```python
from build123d import *

# Parameters (mm, degrees)
SKETCH2_R               = 18
BOSS_EXTRUDE1_DEPTH     = 60
BOSS_EXTRUDE2_DEPTH     = 53
BOSS_EXTRUDE3_DEPTH     = 2
CUT_EXTRUDE3_DEPTH      = 97.822001632
CUT_EXTRUDE3_DEPTH_BACK = 97.822001632
BOSS_EXTRUDE4_START     = -56
SKETCH6_R               = 18
BOSS_EXTRUDE4_DEPTH     = 56
SKETCH8_R               = 3.017040472
BOSS_EXTRUDE5_DEPTH     = 10
SKETCH9_R               = 40
BOSS_EXTRUDE6_DEPTH     = 4.2
CUT_EXTRUDE4_DEPTH      = 104.317471969
CIRPATTERN1_COUNT       = 3


with BuildPart() as part:
    # Sketch2 → Boss-Extrude1 (new body)
    with BuildSketch(Plane.XY):
        Circle(SKETCH2_R)
    extrude(amount=BOSS_EXTRUDE1_DEPTH)

    # Sketch3 → Boss-Extrude2 (add)
    with BuildSketch(Plane.XY):
        with BuildLine():
            Line((-25.5, 0), (-25.5, 58.5))
            Line((-25.5, 58.5), (25.5, 58.5))
            Line((25.5, 58.5), (25.5, 0))
            ThreePointArc((25.5, 0), (0, -25.5), (-25.5, 0))
        make_face()
    extrude(amount=BOSS_EXTRUDE2_DEPTH)

    # Sketch4 → Boss-Extrude3 (add)
    with BuildSketch(Plane.XY):
        with BuildLine():
            Line((-3.6, 19.027416998), (-19.027416998, 3.6))
            Line((-19.027416998, 3.6), (-44.9, 3.6))
            ThreePointArc((-44.9, 3.6), (-48.5, 0), (-44.9, -3.6))
            Line((-44.9, -3.6), (-19.027416998, -3.6))
            Line((-19.027416998, -3.6), (-3.6, -19.027416998))
            Line((-3.6, -19.027416998), (-3.6, -44.9))
            ThreePointArc((-3.6, -44.9), (0, -48.5), (3.6, -44.9))
            Line((3.6, -44.9), (3.6, -19.027416998))
            Line((3.6, -19.027416998), (19.027416998, -3.6))
            Line((19.027416998, -3.6), (44.9, -3.6))
            ThreePointArc((44.9, -3.6), (48.5, 0), (44.9, 3.6))
            Line((44.9, 3.6), (19.027416998, 3.6))
            Line((19.027416998, 3.6), (3.6, 19.027416998))
            Line((3.6, 19.027416998), (3.6, 44.9))
            ThreePointArc((3.6, 44.9), (0, 48.5), (-3.6, 44.9))
            Line((-3.6, 44.9), (-3.6, 19.027416998))
        make_face()
    extrude(amount=-BOSS_EXTRUDE3_DEPTH)

    # Sketch5 → Cut-Extrude3 (cut, two sides: drawn at the far end of the back side and taken through both)
    with BuildSketch(Plane(origin=(0, 0, 0), x_dir=(0, 0, -1), z_dir=(1, 0, 0)).offset(-CUT_EXTRUDE3_DEPTH_BACK)):
        with BuildLine():
            Line((-53, 14.147312787), (-45.647312787, 14.147312787))
            ThreePointArc((-45.647312787, 14.147312787), (-17.612429059, 2.534883727), (-6, -25.5))
            Line((-6, -25.5), (-53, -25.5))
            Line((-53, -25.5), (-53, 14.147312787))
        make_face()
    extrude(amount=CUT_EXTRUDE3_DEPTH + CUT_EXTRUDE3_DEPTH_BACK, mode=Mode.SUBTRACT)

    # Sketch6 → Boss-Extrude4 (add)
    with BuildSketch(Plane.XY.offset(60).offset(BOSS_EXTRUDE4_START)):
        with Locations(Location((0, 0, 0), (0, 0, 128.190277301))):
            Circle(SKETCH6_R)
    extrude(amount=BOSS_EXTRUDE4_DEPTH)

    # Sketch8 → Boss-Extrude5 (add)
    with BuildSketch(Plane.XY):
        Circle(SKETCH8_R)
    extrude(amount=-BOSS_EXTRUDE5_DEPTH)

    # Sketch9 → Boss-Extrude6 (add)
    with BuildSketch(Plane(origin=(0, 0, -10), x_dir=(-1, 0, 0), z_dir=(0, 0, -1))):
        Circle(SKETCH9_R)
    extrude(amount=BOSS_EXTRUDE6_DEPTH)

    # Sketch11 → Cut-Extrude4 (cut, through all)
    with BuildSketch(Plane.XY.offset(-10)):
        with BuildLine():
            Line((12.5, 0), (30, 0))
            ThreePointArc((30, 0), (19.283628291, 22.981333294), (-5.20944533, 29.54423259))
            Line((-5.20944533, 29.54423259), (-2.170602221, 12.310096913))
            ThreePointArc((-2.170602221, 12.310096913), (8.034845121, 9.575555539), (12.5, 0))
        make_face()
    cut_extrude4 = extrude(amount=-CUT_EXTRUDE4_DEPTH, mode=Mode.SUBTRACT)

    # CirPattern1: Cut-Extrude4 ×3 about axis
    cirpattern1_axis = Axis((0, 0, 0), (0, 0, 1))
    for i in range(1, CIRPATTERN1_COUNT):
        add(cut_extrude4.rotate(cirpattern1_axis, i * 360 / CIRPATTERN1_COUNT), mode=Mode.SUBTRACT)


solid = part.part
```
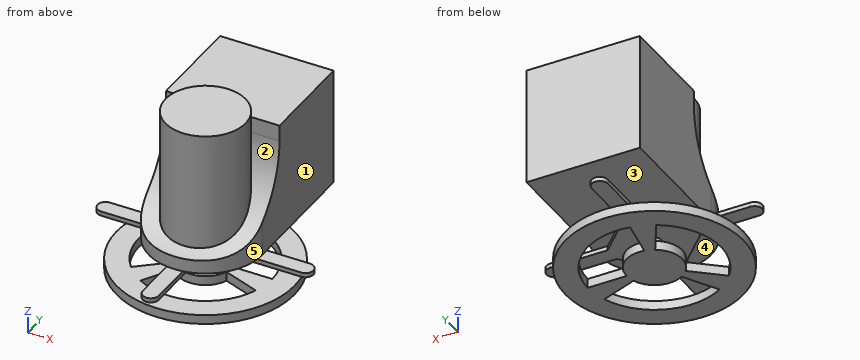
Design review of the part built by this model. Coordinates are the model's own, in mm. Face numbers are marked on the shaded views. A direction names the side the tool comes from. Coordinates: 2 decimals unless noted, no trailing zeros. Order: outer loops, then holes, each group sorted by start corner. A loop starts at its lowest first (then second) coordinate and runs counter-clockwise, first axis right, second up. Notation, with made-up numbers: M -34.5,51 L 14.5,51 A19 ccw 14.5,79 Z; hole C 62,66.25 d11. An arc over 180 degrees is marked long. Answer as a JSON object with one key per item and string values. Group by question number.
1) Add section D-D, the plane z = 41. Write out the cut boundary in (x, y).
2) Add section A-A, the plane x = 33.5. Write out the cut boundary in (y, z).
3) Add section C-C, the plane x = 23. Write out the cut boundary in (y, z), then the cut area to 3 significant figures.
4) For pin 1 (2 mm diameter, centred on x = -26, z = -1, fed in from +Y); pin 2 (16 mm diameter, centred on y = 34.5, z = 16, fed in from -X); pin 3 (4 mm diameter, centred on x = -20, y = 18, fed in from -Z), all flat-tipped, find the tip position at first contact; note any pin that passes through.
5) Wall thickness on L1, parallel to Y at x = 16.5, z = 30.5; L2, parallel to Z at x = -5, y = 6; L3, parallel to Y at x = -19, z = -1: over which ranges is each line inside the solid? List them lowest first.
6) Add section B-B, the plane z = 49. Write out the cut boundary in (x, y).
7) Tool access review of the marked faces 1, 2, 3, 4 and 5: name each direction out of +Z, -Z, +X, -X, +Y, -Y from which nothing blocks a thin tool from reaching the whole face with its end or side.
Computed values:
{
 "1": {"outline": "M -25.5,13.87 L -11.47,13.87 A18 ccw long 11.47,13.87 L 25.5,13.87 L 25.5,58.5 L -25.5,58.5 Z"},
 "2": {"outline": "M -21.86,-14.2 L 21.86,-14.2 L 21.86,-10 L -21.86,-10 Z; M -3.6,-2 L 3.6,-2 L 3.6,0 L -3.6,0 Z"},
 "3": {"outline": "M -32.73,-14.2 L -19.26,-14.2 L -19.26,-10 L -32.73,-10 Z; M -11.01,0 L -3.6,0 L -3.6,-2 L 3.6,-2 L 3.6,0 L 58.5,0 L 58.5,53 L 14.15,53 L 14.15,45.65 A39.65 cw -11.01,8.74 Z; M -8.37,-14.2 L 0,-14.2 L 0,-10 L -8.37,-10 Z; M 19.26,-14.2 L 32.73,-14.2 L 32.73,-10 L 19.26,-10 Z", "area": "2,990 mm^2"},
 "4": {"pin 1": "stops at y = 3.6", "pin 2": "stops at x = -25.5", "pin 3": "stops at z = 0"},
 "5": {"L1": "y = -7.19 to 7.19, 11.14 to 58.5", "L2": "z = -14.2 to -10, -2 to 60", "L3": "y = -3.63 to 3.63"},
 "6": {"outline": "M -25.5,14.15 L -11.13,14.15 A18 ccw long 11.13,14.15 L 25.5,14.15 L 25.5,58.5 L -25.5,58.5 Z"},
 "7": {"face 1": "+Z, +X, +Y, -Y", "face 2": "+Z", "face 3": "+Y", "face 4": "-X, -Y", "face 5": "+Z, -Y"}
}
